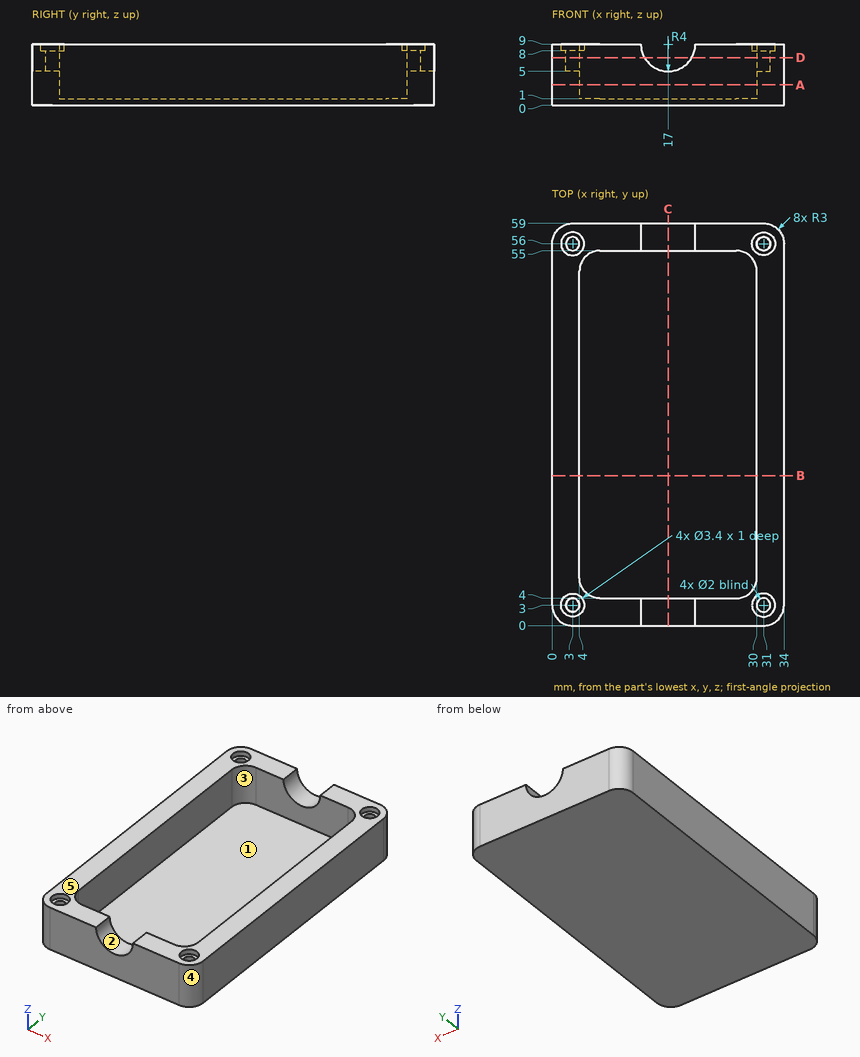
Study the drawing (mm; zero at the part's minimum x, y, z) and answer. A direction names the side the tool comes from. Round coordinates to 2 decimals unless told otherwise and drop trailing zeros. Write each loop counter-clockwise with the first axis right and the second up, starting at its lowest first coordinate (ties: lowest second). Pieces come first, ordered by that corner, then holes. Notation, with made-up numbers: (-1.5, -37) - (43.5, -37) arc R21 cw to (43.5, -9) - close; hole circle Ø9 at (-34, -18.5). An arc over 180 degrees is marked (long way). Use a Markdown table: item, result. Add a question column.
1. Flat-ended cylindrical pins translate along their axes: P1, Ø3, axis at x = 14.5, y = 47, coming from the +Z side; P2, Ø0.6, axis at x = 31, y = 56, coming from the +Z side; P3, Ø2.5, axis at x = 3, y = 3, coming from the +Z side. Find the tip coordinate at first contact, or state that the pin passes through.
2. The part is cut by section D-D (z = 7). Write down the section's boundary in (x, y), and give its area (3 significant figures).
3. Consider line 1 (Y direction, x = 3, z = 6.2); line 2 (X direction, y = 31, z = 4); line 3 (Y direction, x = 3, z = 8.8). Determine where each line is inside the solid, lowest interval first.
4. The part is cut by section C-C (x = 17). Write down the section's boundary in (y, z), and give its area (3 significant figures).
5. The part is cut by section B-B (y = 22). Write down the section's boundary in (x, z).
6. A tool of negligible diameter and unlimited length cuts with its end or side. For the marked faces 1 and 2, from which of +Z, -Z, +X, -X, +Y, -Y can it reach the whole face along a straight path? Write none if from no direction.
7. For a pull along X with two mould halves and no side action, classify the marked faces 3, 4 and 5 as +X half, -X half, draft (parallel to the pull), parting line (faces both ways), or undercut.
8. The part is cut by section A-A (z = 3). Write down the section's boundary in (x, y).
Reported:
| question | item | result |
|---|---|---|
| 1 | P1 | z = 1 |
| 1 | P2 | z = 5 |
| 1 | P3 | z = 8 |
| 2 | outline | (0, 3) arc R3 ccw to (3, 0) - (13.54, 0) - (13.54, 4) - (7, 4) arc R3 cw to (4, 7) - (4, 52) arc R3 cw to (7, 55) - (13.54, 55) - (13.54, 59) - (3, 59) arc R3 ccw to (0, 56) - close; (20.46, 0) - (31, 0) arc R3 ccw to (34, 3) - (34, 56) arc R3 ccw to (31, 59) - (20.46, 59) - (20.46, 55) - (27, 55) arc R3 cw to (30, 52) - (30, 7) arc R3 cw to (27, 4) - (20.46, 4) - close; hole circle Ø2 at (3, 3); hole circle Ø2 at (3, 56); hole circle Ø2 at (31, 3); hole circle Ø2 at (31, 56) |
| 2 | area | 612 mm^2 |
| 3 | line 1 | 0 to 2, 4 to 55, 57 to 59 |
| 3 | line 2 | 0 to 4, 30 to 34 |
| 3 | line 3 | 0 to 1.3, 4.7 to 54.3, 57.7 to 59 |
| 4 | outline | (0, 0) - (59, 0) - (59, 5) - (55, 5) - (55, 1) - (4, 1) - (4, 5) - (0, 5) - close |
| 4 | area | 91.0 mm^2 |
| 5 | outline | (0, 0) - (34, 0) - (34, 9) - (30, 9) - (30, 1) - (4, 1) - (4, 9) - (0, 9) - close |
| 6 | face 1 | +Z |
| 6 | face 2 | +Z, +Y, -Y |
| 7 | face 3 | undercut |
| 7 | face 4 | +X half |
| 7 | face 5 | draft |
| 8 | outline | (0, 3) arc R3 ccw to (3, 0) - (31, 0) arc R3 ccw to (34, 3) - (34, 56) arc R3 ccw to (31, 59) - (3, 59) arc R3 ccw to (0, 56) - close; hole (4, 7) arc R3 ccw to (7, 4) - (27, 4) arc R3 ccw to (30, 7) - (30, 52) arc R3 ccw to (27, 55) - (7, 55) arc R3 ccw to (4, 52) - close |
